Check sheet for the modelled part. Datum: model origin and axes. Units: mm. A direction names the side the tool comes from. Give positions to 0.01 mm unless a question says otherwise; leave off trailing zeros. Write each loop counter-clockwise with the first axis right and the second up, starting at its lowest first coordinate (ties: lowest second). Pieces come first, ordered by that corner, then holes. Notation, with made-up numbers: M 30,-24.75 L 70,-24.75 A25 ccw 70,-11.75 Z; hole C 37,11 d4. An arc over 180 degrees is marked long. Write each question's results on one line, items separated by ' | '. Start each with the question number.
from build123d import *

# Parameters (mm, degrees)
F0_W     = 67.18
F0_H     = 138.35
F1_DEPTH = 7.2
F2_R     = 9.4
F3_R     = 3.2
F4_R     = 3.6
F5_DEPTH = 0.76
F6_SIZE  = 0.33


with BuildPart() as f1:
    # F0 (on Top) → F1 (new body)
    with BuildSketch(Plane.XY):
        Rectangle(F0_W, F0_H)
    extrude(amount=F1_DEPTH)

    # F2
    f2_edges = [f1.edges().sort_by_distance(p)[0] for p in [
        (33.59, 69.175, 3.6),
        (-33.59, 69.175, 3.6),
        (-33.59, -69.175, 3.6),
        (33.59, -69.175, 3.6),
    ]]
    fillet(f2_edges, radius=F2_R)

    # F3
    f3_edges = [f1.edges().sort_by_distance(p)[0] for p in [
        (33.59, 0, 0),
        (33.59, 0, 7.2),
    ]]
    fillet(f3_edges, radius=F3_R)

    # F4 (on face) → F5 (join)
    with BuildSketch(Plane(origin=(0, 0, 0), x_dir=(1, 0, 0), z_dir=(0, 0, -1))):
        with Locations((20.27, -62.235)):
            Circle(F4_R)
    extrude(amount=F5_DEPTH)

    # F6
    f6_edges = [f1.edges().sort_by_distance(p)[0] for p in [
        (16.67, 62.235, -0.76),
    ]]
    chamfer(f6_edges, length=F6_SIZE)


solid = f1.part
Q1. Section check A-A on x = -2. Record the boundary of the cut face in (y, z) (3 decimals).
Q2. Section check B-B on y = 51.5. Record the boundary of the cut face in (x, z), plus the area to 3 significant figures.
Q3. Scan lines: L1, parallel to Z at x = 18, y = 24.5; L2, parallel to X at y = -32, z = 3; L3, parallel to Y at x = -4, z = 5.75. Record each from-to range of solid material in increasing order.
Q4. Depth check by flat-ended pin: pin 1 Ø18 at (x, y) = (0, -2) entering from -Z; pin 2 Ø1.5 at (y, z) = (-40, 0.5) entering from -X. Enter the tip coordinate at first touch or a pass-through.
Q5. Tool access check on faces 1 (the face through (23.6, 63.6, -0.2)), 2 (the face through (-0.3, 68.2, 6.3)). Record the directions out of +Z, -Z, +X, -X, +Y, -Y that give a thin tool (end or side, any length) a straight path to the whole face; none if there is none.
Q6. Section check C-C on x = 20.27. Record the boundary of the cut face in (y, z) (3 decimals).
Check result:
1) outline: M -69.175,3.2 A3.2 ccw -65.975,0 L 65.975,0 A3.2 ccw 69.175,3.2 L 69.175,4 A3.2 ccw 65.975,7.2 L -65.975,7.2 A3.2 ccw -69.175,4 Z
2) outline: M -33.59,3.2 A3.2 ccw -30.39,0 L 30.39,0 A3.2 ccw 33.59,3.2 L 33.59,4 A3.2 ccw 30.39,7.2 L -30.39,7.2 A3.2 ccw -33.59,4 Z | area: 475 mm^2
3) L1: 0 to 7.2 | L2: -33.58 to 33.58 | L3: -68.65 to 68.65
4) pin 1: z = 0 | pin 2: x = -32.93
5) face 1: -Z | face 2: +Z, +X, -X, +Y
6) outline: M -69.175,3.2 A3.2 ccw -65.975,0 L 58.635,0 L 58.635,-0.43 L 58.965,-0.76 L 65.505,-0.76 L 65.835,-0.43 L 65.835,0 L 65.975,0 A3.2 ccw 69.175,3.2 L 69.175,4 A3.2 ccw 65.975,7.2 L -65.975,7.2 A3.2 ccw -69.175,4 Z
